from build123d import *

# Parameters (mm, degrees)
F1_DEPTH    = 3.81
F2_W        = 9.0688861602
F2_H        = 3.81
F3_DEPTH    = 6.35
F4_SIZE     = 1.27
F5_W        = 9.0688861602
F5_H        = 3.81
F6_DEPTH    = 5.08
F7_T1_DEPTH = 35.1971853179
F8_R        = 0.9525
F9_DEPTH    = 8.89


# Not quite as in the source:
# - a fillet or chamfer that OpenCascade refuses, or shapes differently, is made with other operations: its cross-section is extruded or revolved along the edge and cut away or added


with BuildPart() as f1:
    # F0 (on Top) → F1 (new body)
    with BuildSketch(Plane.XY):
        with BuildLine():
            Line((4.5344430801, -2.4189800566), (-4.5344430801, -2.4189800566))
            ThreePointArc((-4.5344430801, -2.4189800566), (-11.6244136954, -22.8629027748), (-4.5344430801, -43.306825493))
            Line((-4.5344430801, -43.306825493), (4.5344430801, -43.306825493))
            ThreePointArc((4.5344430801, -43.306825493), (11.6244136954, -22.8629027748), (4.5344430801, -2.4189800566))
        make_face()
    extrude(amount=F1_DEPTH)

    # F2 (on face) → F3 (join)
    with BuildSketch(Plane(origin=(0, -2.4189800566, 0), x_dir=(-1, 0, 0), z_dir=(0, 1, 0))):
        with Locations((0, 1.905)):
            Rectangle(F2_W, F2_H)
    extrude(amount=F3_DEPTH)

    # F4
    f4_edges = [f1.edges().sort_by_distance(p)[0] for p in [
        (0, 3.93102, 0),
    ]]
    chamfer(f4_edges, length=F4_SIZE)

    # F5 (on face) → F6 (join)
    with BuildSketch(Plane.XZ.offset(43.306825493)):
        with Locations((0, 1.905)):
            Rectangle(F5_W, F5_H)
    extrude(amount=F6_DEPTH)

    # F7: chamfer of 5.08 on 1 edges, made by hand

    # F7_s2 → F7_t1 (cut)
    with BuildSketch(Plane.YZ.offset(-17.598592659)):
        Polygon((-43.306825493, 0), (-48.386825493, 5.08), (-48.386825493, 0), align=None)
    extrude(amount=F7_T1_DEPTH, mode=Mode.SUBTRACT)

    # F8 (on face) → F9 (cut)
    with BuildSketch(Plane(origin=(0, 3.9310199434, 0), x_dir=(-1, 0, 0), z_dir=(0, 1, 0))):
        with Locations((0, 2.4971892126)):
            Circle(F8_R)
    extrude(amount=-F9_DEPTH, mode=Mode.SUBTRACT)


solid = f1.part
Model file for the job. Use its own axes, mm. A direction names the side the tool comes from. Give positions to 0.01 mm unless a question says otherwise; leave off trailing zeros. Write each loop counter-clockwise with the first axis right and the second up, starting at its lowest first coordinate (ties: lowest second). Pieces come first, ordered by that corner, then holes. Notation, with made-up numbers: (-25.75, 33) -> (-13.75, 33) arc R17 ccw to (-13.75, 57) -> close; hole circle Ø8 at (1, 46.5). An arc over 180 degrees is marked (long way). Write item = value, one per line.
(1) Slice it at A-A, the plane x = 0. Give the cut face in (y, z).
Determined:
outline = (-47.12, 3.81) -> (-43.31, 0) -> (2.66, 0) -> (3.93, 1.27) -> (3.93, 1.54) -> (-4.96, 1.54) -> (-4.96, 3.45) -> (3.93, 3.45) -> (3.93, 3.81) -> close
(2) Probe line 1 along Z through (x, y) = (0, 0.25); line 2 along X through (y, z) = (0, 1.2); line 3 along X through (y, z) = (-19.5, 1.9). List the from-to ranges inside material, lowest first.
Determined:
line_1 = 0 to 1.54, 3.45 to 3.81
line_2 = -4.53 to 4.53
line_3 = -11.45 to 11.45
(3) Mould opens along X. For faces 4 (the face through (-4.534, 1, 2)), 5 (the face through (0, -4.959, 3)), 6 (the face through (0.124, -0.452, 3.442)), 7 (the face through (4.534, -44, 3)) say: released by +X, released by -X, zero draft, split by the parting line, or undercut.
Determined:
face_4 = released by -X
face_5 = undercut
face_6 = undercut
face_7 = released by +X
(4) Flat gauge pins, fed straight in: P1, Ø0.6, axis at x = 0, z = 3, coming from the +Y side; P2, Ø1.1, axis at y = -44.5, z = 2, coming from the +X side. Where does each tip first touch, or does it go through?
Determined:
P1 = -4.96
P2 = 4.53
(5) Slice it at C-C, the plane y = -18. Give the cut face in (x, z).
Determined:
outline = (-11.26, 0) -> (11.26, 0) -> (11.26, 3.81) -> (-11.26, 3.81) -> close
(6) Slice it at B-B, the plane z = 0.8. Give the cut face in (x, y), then the cut area to 3 significant figures.
Determined:
outline = (-4.53, -44.11) -> (4.53, -44.11) -> (4.53, -43.31) arc R33.02 ccw to (4.53, -2.42) -> (4.53, 3.46) -> (-4.53, 3.46) -> (-4.53, -2.42) arc R33.02 ccw to (-4.53, -43.31) -> close
area = 827 mm2
(7) Tool access for faces 1 (the face through (-4.534, -44, 3)), 2 (the face through (0, -21, 3.81)), 3 (the face through (4.534, 1, 2)): list every direction of +Z, -Z, +X, -X, +Y, -Y with a clear straight run to the whole face (end or side of a thin tool).
Determined:
face_1 = +Z, -Z, -X, -Y
face_2 = +Z, +X, -X, +Y, -Y
face_3 = +Z, -Z, +X, +Y
(8) Slice it at D-D, the plane x = -7. Give the cut face in (y, z), then the cut area to 3 significant figures.
Determined:
outline = (-39.72, 0) -> (-6.01, 0) -> (-6.01, 3.81) -> (-39.72, 3.81) -> close
area = 128 mm2
